Could you check a few things on this model? Use its own coordinates, in mm. Face numbers are marked on the shaded views. A direction names the side the tool comes from. Give positions to 0.01 mm unless a question says otherwise; leave off trailing zeros. Loops run counter-clockwise (first coordinate to the right, second up) from the corner with the lowest first, then second, coordinate; pieces in that order, holes last. Notation, with made-up numbers: M 29.25,-4 L 36.25,-4 A27 ccw 36.25,28 Z; hole C 89.5,66 d1. An arc over 180 degrees is marked long. Write each question's results on one line, items separated by ' | '. Start each with the question number.
from build123d import *

# Parameters (mm, degrees)
SKETCH1_W           = 35
SKETCH1_H           = 80
BOSS_EXTRUDE1_DEPTH = 20
BOSS_EXTRUDE2_DEPTH = 10
SKETCH3_W           = 6
SKETCH3_H           = 6
CUT_EXTRUDE2_DEPTH  = 39.37
SKETCH6_W           = 4
SKETCH6_H           = 5
CUT_EXTRUDE4_DEPTH  = 5
SKETCH7_W           = 29
SKETCH7_H           = 74
CUT_EXTRUDE5_DEPTH  = 16
SKETCH11_W          = 12.542842321
SKETCH11_H          = 6
CUT_EXTRUDE8_DEPTH  = 16
BOSS_EXTRUDE3_DEPTH = 10
FILLET5_R           = 2.2
SKETCH13_W          = 7
SKETCH13_H          = 18
BOSS_EXTRUDE4_DEPTH = 8
SKETCH14_W          = 2
SKETCH14_H          = 12.5
CUT_EXTRUDE9_DEPTH  = 54.114593098
SKETCH15_W          = 2
SKETCH15_H          = 12.5
CUT_EXTRUDE10_DEPTH = 54.114593098
SKETCH16_W          = 16
SKETCH16_H          = 6
CUT_EXTRUDE11_DEPTH = 10
SKETCH17_W          = 16
SKETCH17_H          = 6
BOSS_EXTRUDE5_DEPTH = 2
SKETCH18_W          = 6
SKETCH18_H          = 6
CUT_EXTRUDE12_DEPTH = 19
SKETCH19_R          = 1
CUT_EXTRUDE13_DEPTH = 3


with BuildPart() as part:
    # Sketch1 → Boss-Extrude1 (new body)
    with BuildSketch(Plane.XY):
        Rectangle(SKETCH1_W, SKETCH1_H)
    extrude(amount=BOSS_EXTRUDE1_DEPTH)

    # Sketch7 → Cut-Extrude5 (cut)
    with BuildSketch(Plane.XY.offset(20)):
        Rectangle(SKETCH7_W, SKETCH7_H)
    extrude(amount=-CUT_EXTRUDE5_DEPTH, mode=Mode.SUBTRACT)



with BuildPart() as body_2:
    # Sketch2 → Boss-Extrude2 (new body)
    with BuildSketch(Plane(origin=(17.5, 0, 0), x_dir=(0, 0, -1), z_dir=(1, 0, 0))):
        Polygon((0, 5), (25.4, 5), (25.4, -5), (0, -5), (-20, -5), (-20, 5), align=None)
    extrude(amount=BOSS_EXTRUDE2_DEPTH)

    # Sketch3 → Cut-Extrude2 (cut)
    with BuildSketch(Plane.XY.offset(20)):
        with Locations((22.5, 0)):
            Rectangle(SKETCH3_W, SKETCH3_H)
    extrude(amount=-CUT_EXTRUDE2_DEPTH, mode=Mode.SUBTRACT)

    # Sketch6 → Cut-Extrude4 (cut)
    with BuildSketch(Plane(origin=(27.5, 0, 0), x_dir=(0, 0, -1), z_dir=(1, 0, 0))):
        with Locations((21.230369208, 0)):
            Rectangle(SKETCH6_W, SKETCH6_H)
    extrude(amount=-CUT_EXTRUDE4_DEPTH, mode=Mode.SUBTRACT)

    # Sketch11 → Cut-Extrude8 (cut)
    with BuildSketch(Plane.XY.offset(20)):
        with Locations((25.771421161, 0)):
            Rectangle(SKETCH11_W, SKETCH11_H)
    extrude(amount=-CUT_EXTRUDE8_DEPTH, mode=Mode.SUBTRACT)


with BuildPart() as part_1:
    add(part.part)

    add(body_2.part)  # Boss-Extrude3 merges body 2
    # Sketch12 → Boss-Extrude3 (add)
    with BuildSketch(Plane.XZ.offset(5)):
        with BuildLine():
            Line((26.553770823, 0), (17.5, 0))
            Line((17.5, 0), (17.5, -4.56807309))
            ThreePointArc((17.5, -4.56807309), (24.455433698, -7.097339482), (26.553770823, 0))
        make_face()
    extrude(amount=-BOSS_EXTRUDE3_DEPTH)

    # Fillet5
    fillet5_edges = [part_1.edges().sort_by_distance(p)[0] for p in [
        (22.5, 0, -19.37),
    ]]
    fillet(fillet5_edges, radius=FILLET5_R)

    # Sketch13 → Boss-Extrude4 (add)
    with BuildSketch(Plane(origin=(0, 0, 0), x_dir=(-1, 0, 0), z_dir=(0, 0, -1))):
        with Locations((0, 20)):
            Rectangle(SKETCH13_W, SKETCH13_H)
        with Locations((0, -20)):
            Rectangle(SKETCH13_W, SKETCH13_H)
    extrude(amount=BOSS_EXTRUDE4_DEPTH)

    # Sketch14 → Cut-Extrude9 (cut, through all)
    with BuildSketch(Plane(origin=(3.5, 0, 0), x_dir=(0, 0, -1), z_dir=(1, 0, 0))):
        with Locations((4.000507047, 20.000395676)):
            Rectangle(SKETCH14_W, SKETCH14_H)
    extrude(amount=-CUT_EXTRUDE9_DEPTH, mode=Mode.SUBTRACT)

    # Sketch15 → Cut-Extrude10 (cut, through all)
    with BuildSketch(Plane(origin=(3.5, 0, 0), x_dir=(0, 0, -1), z_dir=(1, 0, 0))):
        with Locations((3.99995913, -20.00010798)):
            Rectangle(SKETCH15_W, SKETCH15_H)
    extrude(amount=-CUT_EXTRUDE10_DEPTH, mode=Mode.SUBTRACT)

    # Sketch16 → Cut-Extrude11 (cut)
    with BuildSketch(Plane(origin=(19.5, 0, 0), x_dir=(0, 0, -1), z_dir=(1, 0, 0))):
        with Locations((-12, 0)):
            Rectangle(SKETCH16_W, SKETCH16_H)
    extrude(amount=-CUT_EXTRUDE11_DEPTH, mode=Mode.SUBTRACT)

    # Sketch17 → Boss-Extrude5 (add)
    with BuildSketch(Plane.ZY.offset(-25.5)):
        with Locations((12, 0)):
            Rectangle(SKETCH17_W, SKETCH17_H)
    extrude(amount=-BOSS_EXTRUDE5_DEPTH)

    # Sketch18 → Cut-Extrude12 (cut)
    with BuildSketch(Plane.XY):
        with Locations((22.5, 0)):
            Rectangle(SKETCH18_W, SKETCH18_H)
    extrude(amount=-CUT_EXTRUDE12_DEPTH, mode=Mode.SUBTRACT)

    # Sketch19 → Cut-Extrude13 (cut)
    with BuildSketch(Plane.XY.offset(20)):
        with Locations((16, 38.5)):
            Circle(SKETCH19_R)
        with Locations((-16, 38.5)):
            Circle(SKETCH19_R)
        with Locations((16, -38.5)):
            Circle(SKETCH19_R)
        with Locations((-16, -38.5)):
            Circle(SKETCH19_R)
    extrude(amount=-CUT_EXTRUDE13_DEPTH, mode=Mode.SUBTRACT)


solid = part_1.part
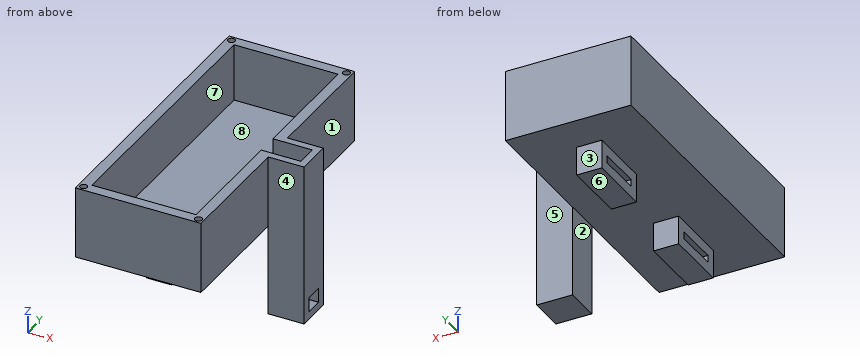
1) If we section it at C-C on z = 6: Write out the boundary of the cut face in (x, y).
2) If we section it at B-B on y = 24: Write out the boundary of the cut face in (x, z).
3) If we section it at A-A on x = -1: Write out the boundary of the cut face in (y, z), plus the area to 3 significant figures.
4) If we section it at D-D on y = -38.5: Write out the boundary of the cut face in (x, z), plus the area to 3 significant figures.
5) Which directions (+Z, -Z, +X, -X, +Y, -Y) give clear straight access to the entire face, cutting with the end or side of a thin tool? Please do the marked faces 1, 2, 3 and 4.
6) Please list where these lines run through material, in increasing order: line 1 (Y direction, x = 16, z = 18.5); line 2 (Y direction, x = -16, z = 17.6); line 3 (X direction, y = 20, z = 11.5). Write a range as from..to.
7) Thinking about a two-plate mould opening in Y: for the marked faces 5, 6, 7 and 8, which applies, pulls with the +Y half, pulls with the -Y half, needs draft (parallel to the pull), parting line crosses it, or undercut?
8) I'm going to push flat-ended pins straight in: P1, Ø4, axis at x = 21.5, z = 6, coming from the +Y side; P2, Ø6.5, axis at y = 22, z = -2, coming from the -X side; P3, Ø9, axis at y = -21, z = -3, coming from the +X side; P4, Ø1, axis at x = 15, y = -20, coming from the -Z side. Where does each tip first touch, or does it pass through?
Calculated:
1) outline: M -17.5,-40 L 17.5,-40 L 17.5,-5 L 27.5,-5 L 27.5,5 L 17.5,5 L 17.5,40 L -17.5,40 Z; hole M -14.5,-37 L 14.5,-37 L 14.5,-3 L 25.5,-3 L 25.5,3 L 14.5,3 L 14.5,37 L -14.5,37 Z
2) outline: M -17.5,0 L -3.5,0 L -3.5,-3 L 3.5,-3 L 3.5,0 L 17.5,0 L 17.5,20 L 14.5,20 L 14.5,4 L -14.5,4 L -14.5,20 L -17.5,20 Z; M -3.5,-8 L 3.5,-8 L 3.5,-5 L -3.5,-5 Z
3) outline: M -40,0 L -29,0 L -29,-8 L -11,-8 L -11,0 L 11,0 L 11,-8 L 29,-8 L 29,0 L 40,0 L 40,20 L 37,20 L 37,4 L -37,4 L -37,20 L -40,20 Z; hole M -26.25,-5 L -13.75,-5 L -13.75,-3 L -26.25,-3 Z; hole M 13.75,-5 L 26.25,-5 L 26.25,-3 L 13.75,-3 Z | area: 654 mm2
4) outline: M -17.5,0 L 17.5,0 L 17.5,20 L 17,20 L 17,17 L 15,17 L 15,20 L -15,20 L -15,17 L -17,17 L -17,20 L -17.5,20 Z | area: 688 mm2
5) face 1: +Z, -Z, +X, +Y | face 2: -Z, -X, +Y, -Y | face 3: -Z, +X, -X, +Y | face 4: +Z, -Z, +X, -Y
6) line 1: y = -40..-39.5, -37.5..-3, 3..37.5, 39.5..40 | line 2: y = -40..-39.5, -37.5..37.5, 39.5..40 | line 3: x = -17.5..-14.5, 14.5..17.5
7) face 5: pulls with the +Y half | face 6: needs draft | face 7: undercut | face 8: undercut
8) P1: stops at y = 5 | P2: stops at x = -17.5 | P3: stops at x = 17.5 | P4: stops at z = 0
